The drawing under review shows one solid part. Ordinate dimensions are in mm from its lowest x, y, z. A direction names the side the tool comes from. Round coordinates to 2 decimals unless told otherwise and drop trailing zeros. Write each loop counter-clockwise with the first axis right and the second up, starting at its lowest first coordinate (ties: lowest second). Pieces come first, ordered by that corner, then holes. Notation, with made-up numbers: (-21, 49) -> (8, 49) arc R12 cw to (8, 65) -> close; hole circle Ø11 at (-26, 85). An arc over 180 degrees is marked (long way). Answer in a Markdown table with one row per item.
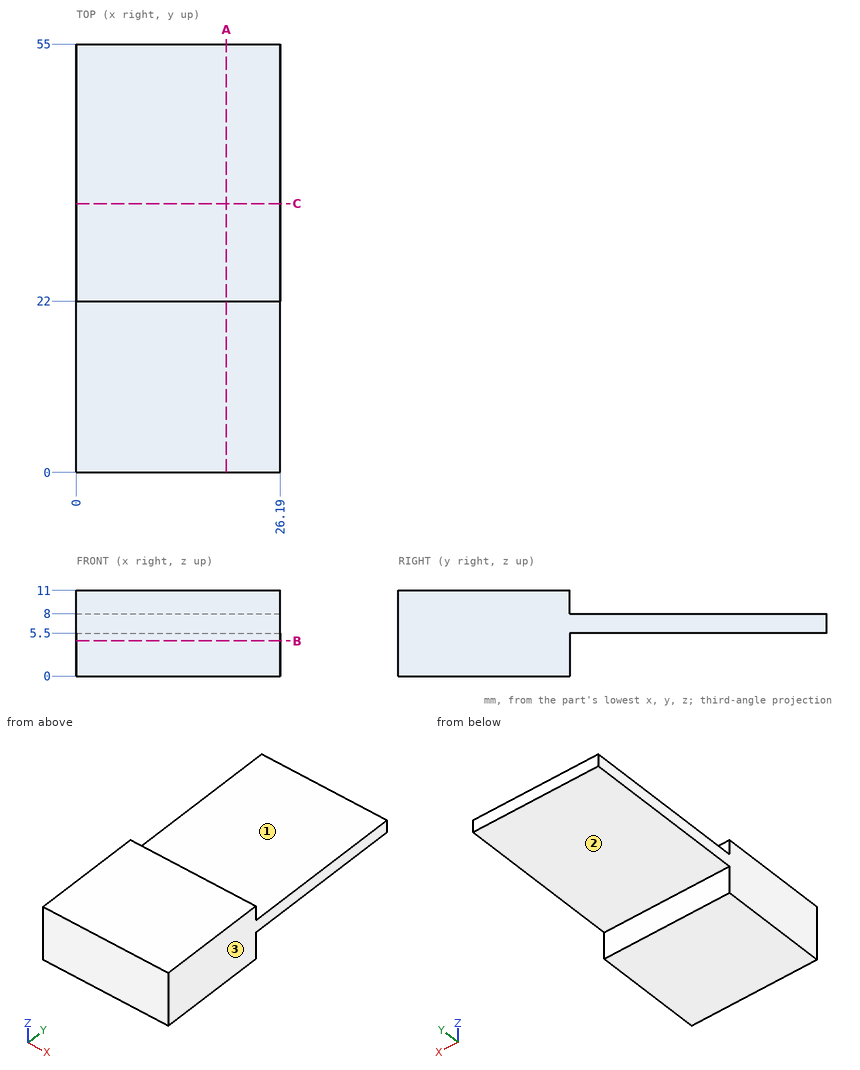
1) Consider section A-A on x = 19.25. State the section outline as (y, z) points.
Solved:
| item | result |
|---|---|
| outline | (0, 0) -> (22, 0) -> (22, 5.5) -> (55, 5.5) -> (55, 8) -> (22, 8) -> (22, 11) -> (0, 11) -> close |
2) For the marked faces 1, 2 and 3, list the 3-axis set-ups (+Z, -Z, +X, -X, +Y, -Y) from which the entire face can be reached by the end or side of a thin tool; tool diameter is ignored.
Solved:
| item | result |
|---|---|
| face 1 | +Z, +X, -X, +Y |
| face 2 | -Z, +X, -X, +Y |
| face 3 | +Z, -Z, +X, +Y, -Y |
3) For line 1 (Z direction, x = 12, y = 45.5); line 2 (Y direction, x = 22.5, z = 3.25), list the stretches that pass through material, from the lowest coordinate up. Write a range as [from, to].
Solved:
| item | result |
|---|---|
| line 1 | [5.5, 8] |
| line 2 | [0, 22] |
4) Clearance check with flat-ended pins moving along their axes: pin 1 Ø12 at (x, y) = (8, 33) entering from -Z; pin 2 Ø4 at (x, z) = (3.5, 5) entering from -Y; pin 3 Ø3 at (x, y) = (21, 28.5) entering from +Z; pin 4 Ø1.6 at (x, z) = (13, 3.5) entering from +Y. State where each tip first meets the part, or that it passes through.
Solved:
| item | result |
|---|---|
| pin 1 | z = 5.5 |
| pin 2 | y = 0 |
| pin 3 | z = 8 |
| pin 4 | y = 22 |
5) Consider section C-C on y = 34.5. State the section outline as (x, z) points.
Solved:
| item | result |
|---|---|
| outline | (0, 5.5) -> (26.19, 5.5) -> (26.19, 8) -> (0, 8) -> close |
6) Consider section B-B on z = 4.5. State the section outline as (x, y) points.
Solved:
| item | result |
|---|---|
| outline | (0, 0) -> (26.19, 0) -> (26.19, 22) -> (0, 22) -> close |
